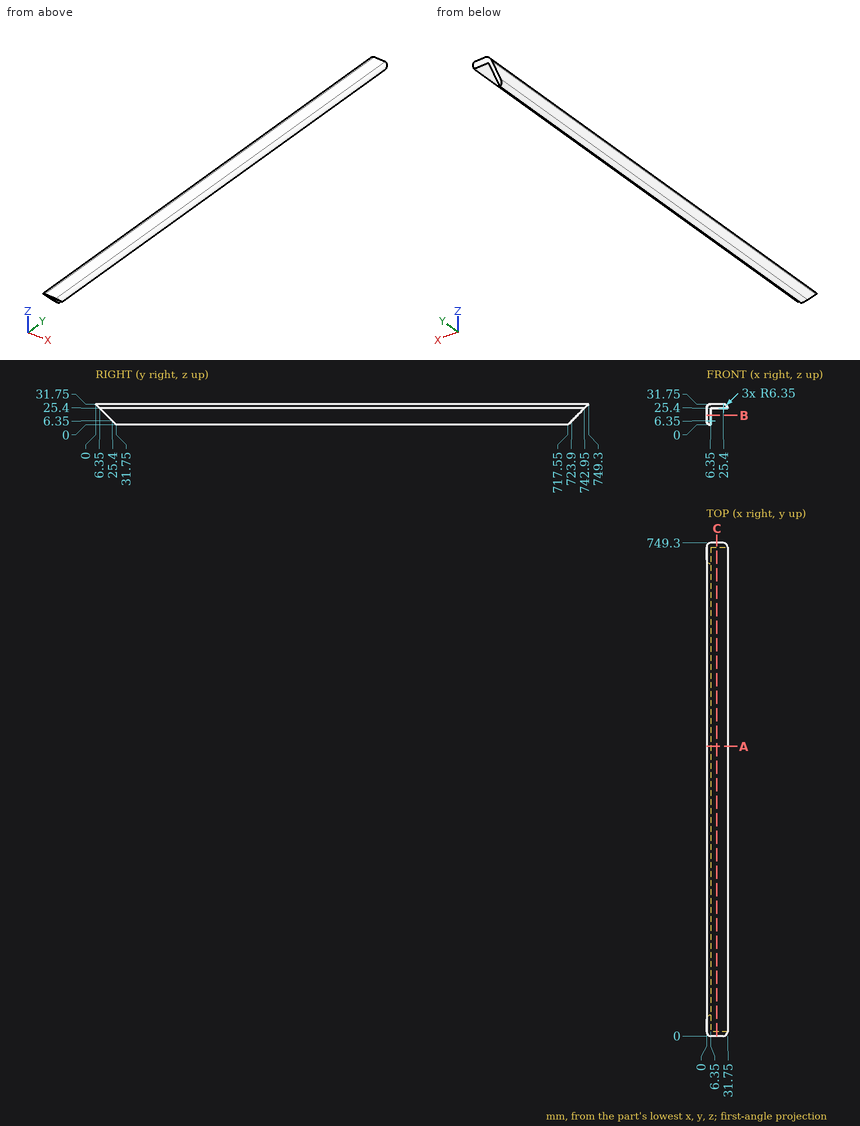
Here's the drawing with two shaded views (mm, measured from the low corner). I have some questions. Coordinates: 2 decimals unless noted, no trailing zeros. Loops run counter-clockwise (first coordinate to the right, second up) from the corner with the lowest first, then second, coordinate; pieces in that order, holes last. Notation, with made-up numbers: M 39.5,61.25 L 91.5,61.25 A12 ccw 91.5,76.25 Z; hole C -6.5,85.25 d3. An arc over 180 degrees is marked long. Put each result on its own line as item: value. Start each with the question number.
(1) Will these pins go through, and if not, where does the flat tip stop? pin 1 Ø1 at (y, z) = (596.5, 16) entering from +X; pin 2 Ø5 at (x, z) = (18, 27) entering from +Y.
(2) Imagine slicing it at C-C on x = 15.5. List the corners of the cut face in (y, z) for me.
(3) Imagine slicing it at B-B on z = 14.5. List the corners of the cut face in (x, y) for me.
(4) Imagine slicing it at A-A on y = 440. List the corners of the cut face in (x, z) for me.
(5) I need wall thicknesses on probe 1 along Z at (x, y) = (24.5, 407.5); probe 2 along X at (y, z) = (110, 20.5); probe 3 along Y at (x, z) = (13, 25.5). Which ranges of each line are inside material? Lowest first, please.
Worked answers:
1. pin 1: stops at x = 6.35
1. pin 2: stops at y = 747.05
2. outline: M 0,31.75 L 6.35,25.4 L 742.95,25.4 L 749.3,31.75 Z
3. outline: M 0,17.25 L 6.35,17.25 L 6.35,732.05 L 0,732.05 Z
4. outline: M 0,6.35 A6.35 ccw 6.35,0 L 6.35,25.4 L 31.75,25.4 A6.35 ccw 25.4,31.75 L 6.35,31.75 A6.35 ccw 0,25.4 Z
5. probe 1: z = 25.4 to 31.75
5. probe 2: x = 0 to 6.35
5. probe 3: y = 6.25 to 743.05
